Build history of the part. All positions in model axes, mm. Round coordinates to 2 decimals unless told otherwise and drop trailing zeros. Write each loop counter-clockwise with the first axis right and the second up, starting at its lowest first coordinate (ties: lowest second). Pieces come first, ordered by that corner, then holes. Notation, with made-up numbers: (62, 13.5) - (113, 13.5) arc R30 cw to (113, 47.5) - close; hole circle Ø7 at (26.25, 49.5). An arc over 180 degrees is marked (long way). One line per question, with ' | ' between items.
from build123d import *

# Parameters (mm, degrees)
F1_DEPTH = 1
F3_D     = 3.5
F5_D     = 6
F6_SIZE  = 0.05


with BuildPart() as f1:
    # F0 (on Top) → F1 (new body)
    with BuildSketch(Plane.XY):
        with BuildLine():
            Line((0, 37.85), (0, 1.5))
            ThreePointArc((0, 1.5), (0.4393398282, 0.4393398282), (1.5, 0))
            Line((1.5, 0), (8, 0))
            ThreePointArc((8, 0), (9.0606601718, 0.4393398282), (9.5, 1.5))
            Line((9.5, 1.5), (9.5, 37.85))
            ThreePointArc((9.5, 37.85), (9.0606601718, 38.9106601718), (8, 39.35))
            Line((8, 39.35), (1.5, 39.35))
            ThreePointArc((1.5, 39.35), (0.4393398282, 38.9106601718), (0, 37.85))
        make_face()
    extrude(amount=-F1_DEPTH)

    # F3 (through all)
    with Locations(Plane.XY):
        with Locations((3.992, 8.943), (3.992, 2.943)):
            Hole(F3_D / 2)

    # F5 (through all)
    with Locations(Plane.XY):
        with Locations((3.969, 23.94), (3.969, 16.937)):
            Hole(F5_D / 2)

    # F6
    f6_edges = [f1.edges().sort_by_distance(p)[0] for p in [
        (9.5, 19.675, 0),
        (0, 19.675, 0),
        (4.75, 0, -1),
        (4.75, 0, 0),
        (9.5, 19.675, -1),
        (4.75, 39.35, 0),
        (0, 19.675, -1),
        (4.75, 39.35, -1),
        (0.43934, 38.91066, 0),
        (0.43934, 38.91066, -1),
        (0.43934, 0.43934, 0),
        (0.43934, 0.43934, -1),
        (9.06066, 38.91066, 0),
        (9.06066, 0.43934, 0),
        (9.06066, 38.91066, -1),
        (9.06066, 0.43934, -1),
    ]]
    chamfer(f6_edges, length=F6_SIZE)


solid = f1.part
Q1. Saw through at B-B, the plane z = -0.75. List the corners of the cut face in (x, y), then the cut area to 3 significant figures.
Found:
outline: (0, 1.5) arc R1.5 ccw to (1.5, 0) - (8, 0) arc R1.5 ccw to (9.5, 1.5) - (9.5, 37.85) arc R1.5 ccw to (8, 39.35) - (1.5, 39.35) arc R1.5 ccw to (0, 37.85) - close; hole circle Ø6 at (3.97, 16.94); hole circle Ø6 at (3.97, 23.94); hole circle Ø3.5 at (3.99, 2.94); hole circle Ø3.5 at (3.99, 8.94) | area: 296 mm^2
Q2. Pull direction X, two halves, no side cores. Call faces 1 (the flat face through (4.8, 39.35, -0.5)), 2 (the cylindrical face through (2.323, 9.469, -0.507)), 3 (the flat face through (9.5, 19.4, -0.5)), 4 (the cylindrical face through (2.36, 19.47, -0.51)): +X half, -X half, draft (parallel to the pull), parting line (faces both ways), or undercut.
Found:
face 1: draft | face 2: undercut | face 3: +X half | face 4: undercut
Q3. Saw through at C-C, the plane y = 16. List the corners of the cut face in (x, z).
Found:
outline: (0, -0.95) - (0.05, -1) - (1.12, -1) - (1.12, 0) - (0.05, 0) - (0, -0.05) - close; (6.82, -1) - (9.45, -1) - (9.5, -0.95) - (9.5, -0.05) - (9.45, 0) - (6.82, 0) - close
Q4. Drop flat-ended pins along their axis: pin 1 (5.5 mm diameter, centred on x = 3.969, y = 16.937, fed in from -Z); pin 2 (4 mm diameter, centred on x = 3.992, y = 2.943, fed in from -Z). Give the stop position or say it passes through.
Found:
pin 1: through | pin 2: z = -1
Q5. Drill centre lines: L1, parallel to Y at x = 4, z = -0.7; L2, parallel to X at y = 3, z = -0.15; L3, parallel to Y at x = 4.25, z = -0.45. Where is each one in solid material? Low to high. Write a range as from..to.
Found:
L1: 0..1.19, 4.69..7.19, 10.69..13.94, 19.94..20.94, 26.94..39.35 | L2: 0..2.24, 5.74..9.5 | L3: 0..1.21, 4.67..7.21, 10.67..13.95, 19.92..20.95, 26.93..39.35
Q6. Saw through at A-A, the plane y = 23.94. List the corners of the cut face in (x, z), then the cut area to 4 significant figures.
Found:
outline: (0, -0.95) - (0.05, -1) - (0.97, -1) - (0.97, 0) - (0.05, 0) - (0, -0.05) - close; (6.97, -1) - (9.45, -1) - (9.5, -0.95) - (9.5, -0.05) - (9.45, 0) - (6.97, 0) - close | area: 3.495 mm^2
